Geometry check sheet. Reference: the model listing, model coordinates, mm. Face numbers are marked on the shaded views. A direction names the side the tool comes from. Coordinates: 2 decimals unless noted, no trailing zeros. Loops run counter-clockwise (first coordinate to the right, second up) from the corner with the lowest first, then second, coordinate; pieces in that order, holes last. Notation, with made-up numbers: (48, 36) - (96, 36) arc R23 cw to (96, 64) - close; hole circle Ø3 at (89.5, -21.75). An arc over 180 degrees is marked (long way). One line per item, written item: value.
from build123d import *

# Parameters (mm, degrees)
SKETCH1_W           = 62
SKETCH1_H           = 35
BOSS_EXTRUDE1_DEPTH = 50
CUT_EXTRUDE3_DEPTH  = 88
SKETCH4_W           = 42
SKETCH4_H           = 20
CUT_EXTRUDE5_DEPTH  = 40
SKETCH5_R           = 1.75
CUT_EXTRUDE7_DEPTH  = 100
CUT_EXTRUDE8_REACH  = 83.664
SKETCH6_R           = 1


with BuildPart() as part:
    # Sketch1 → Boss-Extrude1 (new body)
    with BuildSketch(Plane(origin=(0, 0, 0), x_dir=(1, 0, 0), z_dir=(0, 1, 0))):
        with Locations((31, 17.5)):
            Rectangle(SKETCH1_W, SKETCH1_H)
    extrude(amount=BOSS_EXTRUDE1_DEPTH)

    # Sketch2 → Cut-Extrude3 (cut, through all)
    with BuildSketch(Plane(origin=(62, 0, 0), x_dir=(0, 0, -1), z_dir=(1, 0, 0))):
        Polygon((0, 10), (32, 10), (32, 37), (12, 37), (12, 40), (32, 40), (32, 50), (0, 50), align=None)
    extrude(amount=-CUT_EXTRUDE3_DEPTH, mode=Mode.SUBTRACT)

    # Sketch4 → Cut-Extrude5 (cut)
    with BuildSketch(Plane(origin=(0, 10, 0), x_dir=(1, 0, 0), z_dir=(0, 1, 0))):
        with Locations((31, 22)):
            Rectangle(SKETCH4_W, SKETCH4_H)
    extrude(amount=CUT_EXTRUDE5_DEPTH, mode=Mode.SUBTRACT)

    # Sketch5 → Cut-Extrude7 (cut)
    with BuildSketch(Plane(origin=(0, 10, 0), x_dir=(1, 0, 0), z_dir=(0, 1, 0))):
        with Locations(Location((18, 10, 0), (0, 0, 270))):
            Circle(SKETCH5_R)
        with Locations(Location((44, 10, 0), (0, 0, 270))):
            Circle(SKETCH5_R)
    extrude(amount=-CUT_EXTRUDE7_DEPTH, mode=Mode.SUBTRACT)

    # Sketch6 → Cut-Extrude8 (cut, up to next)
    with BuildSketch(Plane(origin=(0, 40, 0), x_dir=(1, 0, 0), z_dir=(0, 1, 0)), mode=Mode.PRIVATE) as cut_extrude8_sk1:
        with Locations(Location((6, 27, 0), (0, 0, 270))):
            Circle(SKETCH6_R)
    cut_extrude8_tool1 = extrude(cut_extrude8_sk1.sketch, amount=-CUT_EXTRUDE8_REACH, mode=Mode.PRIVATE) & part.part
    # Sketch6 → Cut-Extrude8 (cut, up to next)
    with BuildSketch(Plane(origin=(0, 40, 0), x_dir=(1, 0, 0), z_dir=(0, 1, 0)), mode=Mode.PRIVATE) as cut_extrude8_sk2:
        with Locations(Location((6, 17, 0), (0, 0, 270))):
            Circle(SKETCH6_R)
    cut_extrude8_tool2 = extrude(cut_extrude8_sk2.sketch, amount=-CUT_EXTRUDE8_REACH, mode=Mode.PRIVATE) & part.part
    # Sketch6 → Cut-Extrude8 (cut, up to next)
    with BuildSketch(Plane(origin=(0, 40, 0), x_dir=(1, 0, 0), z_dir=(0, 1, 0)), mode=Mode.PRIVATE) as cut_extrude8_sk3:
        with Locations(Location((56, 17, 0), (0, 0, 270))):
            Circle(SKETCH6_R)
    cut_extrude8_tool3 = extrude(cut_extrude8_sk3.sketch, amount=-CUT_EXTRUDE8_REACH, mode=Mode.PRIVATE) & part.part
    # Sketch6 → Cut-Extrude8 (cut, up to next)
    with BuildSketch(Plane(origin=(0, 40, 0), x_dir=(1, 0, 0), z_dir=(0, 1, 0)), mode=Mode.PRIVATE) as cut_extrude8_sk4:
        with Locations(Location((56, 27, 0), (0, 0, 270))):
            Circle(SKETCH6_R)
    cut_extrude8_tool4 = extrude(cut_extrude8_sk4.sketch, amount=-CUT_EXTRUDE8_REACH, mode=Mode.PRIVATE) & part.part
    add(cut_extrude8_tool1.solids().sort_by_distance((6, 40, -27))[0], mode=Mode.SUBTRACT)
    add(cut_extrude8_tool2.solids().sort_by_distance((6, 40, -17))[0], mode=Mode.SUBTRACT)
    add(cut_extrude8_tool3.solids().sort_by_distance((56, 40, -17))[0], mode=Mode.SUBTRACT)
    add(cut_extrude8_tool4.solids().sort_by_distance((56, 40, -27))[0], mode=Mode.SUBTRACT)


solid = part.part
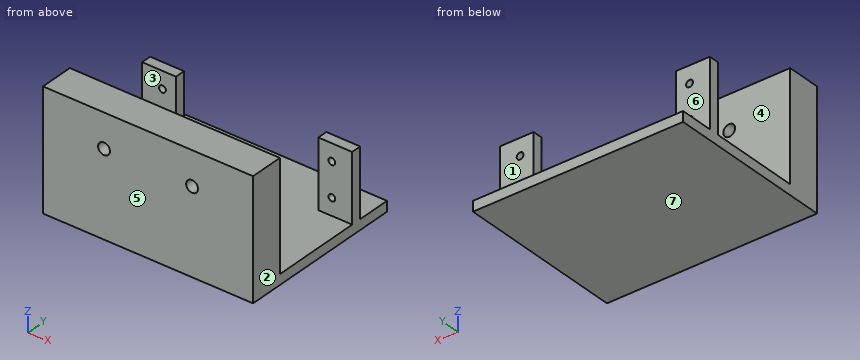
(1) Access from +Z, -Z, +X, -X, +Y, -Y to the whole of each face (thin tool, end or side, straight path). Record for the marked faces 1, 2 and 3.
Reply:
face 1: +Z, +X, -X, +Y
face 2: +Z, -Z, +X, +Y, -Y
face 3: +Z, +X, -X
(2) Cross-section at D-D on z = -27. Record the cut outline in (x, y), and give its area (3 significant figures).
Reply:
outline: (0, 0) - (62, 0) - (62, 10) - (0, 10) - close; (0, 37) - (5, 37) - (5, 40) - (0, 40) - close; (7, 37) - (10, 37) - (10, 40) - (7, 40) - close; (52, 37) - (55, 37) - (55, 40) - (52, 40) - close; (57, 37) - (62, 37) - (62, 40) - (57, 40) - close
area: 668 mm2
(3) Cross-section at B-B on z = -13.5. Record the cut outline in (x, y).
Reply:
outline: (0, 0) - (62, 0) - (62, 10) - (0, 10) - close; (0, 37) - (10, 37) - (10, 40) - (0, 40) - close; (52, 37) - (62, 37) - (62, 40) - (52, 40) - close
(4) Cross-section at C-C on x = 56. Record the cut outline in (y, z), and give its area (3 significant figures).
Reply:
outline: (0, -35) - (50, -35) - (50, -32) - (40, -32) - (40, -28) - (37, -28) - (37, -32) - (10, -32) - (10, 0) - (0, 0) - close; (37, -26) - (40, -26) - (40, -18) - (37, -18) - close; (37, -16) - (40, -16) - (40, -12) - (37, -12) - close
area: 518 mm2
(5) Release check for a two-part mould opening along Y. For the marked faces 4, 5, 6 and 7 record: pulls with the +Y half, pulls with the -Y half, needs draft (parallel to the pull), parting line crosses it, or undercut.
Reply:
face 4: undercut
face 5: pulls with the -Y half
face 6: pulls with the +Y half
face 7: needs draft
(6) Material ranges on probe 1 along X at (y, z) = (37.6, -27); probe 2 along X at (y, z) = (4, -10); probe 3 along Y at (x, z) = (4, -20.5), recorded low to high. Write a range as from..to.
Reply:
probe 1: 0..5, 7..10, 52..55, 57..62
probe 2: 0..16.25, 19.75..42.25, 45.75..62
probe 3: 0..10, 37..40
(7) Cross-section at A-A on x = 18. Record the cut outline in (y, z).
Reply:
outline: (0, -35) - (50, -35) - (50, -32) - (10, -32) - (10, -11.75) - (0, -11.75) - close; (0, -8.25) - (10, -8.25) - (10, 0) - (0, 0) - close
(8) Go/stop test with flat-tipped pins: pin 1 Ø11 at (x, z) = (55.5, -20) entering from -Y; pin 2 Ø2.5 at (x, y) = (56, 38) entering from +Z; pin 3 Ø2.5 at (x, z) = (6, -27) entering from +Y; pin 4 Ø2 at (x, z) = (44, -10) entering from +Y. Record where each tip stops, or that it passes through.
Reply:
pin 1: y = 0
pin 2: z = -12
pin 3: y = 40
pin 4: through
